Autodesk Inventor part; units mm, degrees
ref_plane "YZ Plane" through (0, 0, 0) normal (1, 0, 0) x (0, 1, 0)
ref_plane "XZ Plane" through (0, 0, 0) normal (0, 1, 0) x (-1, 0, 0)
ref_plane "XY Plane" through (0, 0, 0) normal (0, 0, 1) x (1, 0, 0)
sketch "Sketch1" plane through (0, 0, 0) normal (1, 0, 0) x (0, 1, 0)
  line L0 (9.8481, 428.814) -> (120.1519, 448.2635)
  line L1 (131.7365, 440.1519) -> (154.2135, 312.6787)
  line L2 (0, 78.3368) -> (0, 427.0775)
  line L3 (0, 417.0775) -> (0, 78.3368)
  line L4 (503.1119, 189.3047) -> (590.8645, 150.2346)
  line L5 (595.9326, 137.0318) -> (559.5861, 55.3964)
  line L6 (494.9423, 192.942) -> (494.9423, 192.942)
  line L7 (442.0149, 172.9748) -> (165.6696, 297.928)
  arc A0 (442.0149, 172.9748) -> (490.9347, 186.0198) centre (458.495, 209.4221) ccw
  arc A1 (154.2135, 312.6787) -> (165.6696, 297.928) centre (173.9096, 316.1516) ccw
  arc A2 (131.7365, 440.1519) -> (120.1519, 448.2635) centre (121.8884, 438.4154) ccw
  line L8 (9.8481, 428.814) -> (0, 417.0775)
  arc A3 (595.9326, 137.0318) -> (590.8645, 150.2346) centre (586.7972, 141.0991) ccw
  arc A4 (503.1119, 189.3047) -> (490.9347, 186.0198) centre (499.0446, 180.1692) ccw
  line L9 (9.651, 68.3429) -> (550.1017, 49.4699)
  arc A5 (550.1017, 49.4699) -> (559.5861, 55.3964) centre (550.4507, 59.4638) ccw
  arc A6 (0, 78.3368) -> (9.651, 68.3429) centre (10, 78.3368) ccw
  point P0 (0, 0)
  point P1 (0, 0)
  point P2 (130, 450)
  point P3 (156.0472, 302.2788)
  point P4 (0, 0)
  point P5 (534.922, 0)
  point P6 (600, 146.1672)
  point P7 (478.4622, 156.4947)
  point P8 (0, 427.0775)
  point P9 (537.6655, 6.1619)
  point P10 (0, 417.0775)
  dimension "d0" = 130
  dimension "d1" = 404.922
  dimension "d3" = 150
  dimension "d5" = 115
  dimension "d7" = 10
  dimension "d9" = 40
  dimension "d10" = 40
  dimension "d11" = 20
  dimension "d12" = 10
  dimension "d13" = 10
  dimension "d14" = 10
  dimension "d21" = 10
extrude "Extrusion1" add sketch "Sketch1" along normal blind 16
sketch "Sketch2" plane through (0, 0, 0) normal (-1, 0, 0) x (0, 0, 1)
  point P0 (0, 0)
sketch "Sketch3" plane through (0, 0, 0) normal (-1, 0, 0) x (0, 0, 1)
  line L0 (171.0338, 494.9772) -> (173.8576, 488.6347)
  line L1 (166.9664, 504.1126) -> (130.324, 487.7983)
  line L2 (130.324, 487.7983) -> (274.7158, 163.4898)
  line L3 (274.7158, 163.4898) -> (214.4218, 136.6452)
  line L4 (214.4218, 136.6452) -> (218.4892, 127.5097)
  line L5 (218.4892, 127.5097) -> (278.7831, 154.3544)
  line L6 (278.7831, 154.3544) -> (288.9516, 131.5158)
  line L7 (288.9516, 131.5158) -> (298.087, 135.5831)
  line L8 (298.087, 135.5831) -> (143.5268, 482.7303)
  line L9 (143.5268, 482.7303) -> (171.0338, 494.9772)
  line L10 (173.8576, 488.6347) -> (182.9931, 492.702)
  line L11 (182.9931, 492.702) -> (141.0991, 586.7972)
  line L12 (141.0991, 586.7972) -> (131.9637, 582.7298)
  line L13 (301.7603, 135.8301) -> (426.8309, 113.7768)
  line L14 (426.8309, 113.7768) -> (407.5559, 4.4631)
  line L15 (407.5559, 4.4631) -> (417.404, 2.7267)
  line L16 (417.404, 2.7267) -> (438.4154, 121.8884)
  line L17 (438.4154, 121.8884) -> (303.4968, 145.6782)
  line L18 (303.4968, 145.6782) -> (301.7603, 135.8301)
  line L19 (428.814, 9.8481) -> (417.0775, 0)
  line L20 (417.0775, 0) -> (78.3368, 0)
  line L21 (55.3964, 559.5861) -> (137.0318, 595.9326)
  arc A0 (150.2346, 590.8645) -> (137.0318, 595.9326) centre (141.0991, 586.7972) ccw
  line L22 (150.2346, 590.8645) -> (189.3047, 503.1119)
  arc A1 (186.0198, 490.9347) -> (189.3047, 503.1119) centre (180.1692, 499.0446) ccw
  arc A2 (186.0198, 490.9347) -> (172.9748, 442.0149) centre (209.4221, 458.495) ccw
  line L23 (172.9748, 442.0149) -> (297.928, 165.6696)
  arc A3 (297.928, 165.6696) -> (312.6787, 154.2135) centre (316.1516, 173.9096) ccw
  line L24 (312.6787, 154.2135) -> (440.1519, 131.7365)
  arc A4 (448.2635, 120.1519) -> (440.1519, 131.7365) centre (438.4154, 121.8884) ccw
  line L25 (448.2635, 120.1519) -> (428.814, 9.8481)
  line L26 (171.0338, 494.9772) -> (173.8576, 488.6347)
  line L27 (166.9664, 504.1126) -> (130.324, 487.7983)
  line L28 (130.324, 487.7983) -> (274.7158, 163.4898)
  line L29 (274.7158, 163.4898) -> (214.4218, 136.6452)
  line L30 (214.4218, 136.6452) -> (218.4892, 127.5097)
  line L31 (218.4892, 127.5097) -> (278.7831, 154.3544)
  line L32 (278.7831, 154.3544) -> (288.9516, 131.5158)
  line L33 (288.9516, 131.5158) -> (298.087, 135.5831)
  line L34 (298.087, 135.5831) -> (143.5268, 482.7303)
  line L35 (143.5268, 482.7303) -> (171.0338, 494.9772)
  line L36 (173.8576, 488.6347) -> (182.9931, 492.702)
  line L37 (182.9931, 492.702) -> (141.0991, 586.7972)
  line L38 (141.0991, 586.7972) -> (131.9637, 582.7298)
  line L39 (301.7603, 135.8301) -> (426.8309, 113.7768)
  line L40 (426.8309, 113.7768) -> (407.5559, 4.4631)
  line L41 (407.5559, 4.4631) -> (417.404, 2.7267)
  line L42 (417.404, 2.7267) -> (438.4154, 121.8884)
  line L43 (438.4154, 121.8884) -> (303.4968, 145.6782)
  line L44 (303.4968, 145.6782) -> (301.7603, 135.8301)
  line L45 (428.814, 9.8481) -> (417.0775, 0)
  line L46 (417.0775, 0) -> (78.3368, 0)
  line L47 (55.3964, 559.5861) -> (137.0318, 595.9326)
  arc A5 (150.2346, 590.8645) -> (137.0318, 595.9326) centre (141.0991, 586.7972) ccw
  line L48 (150.2346, 590.8645) -> (189.3047, 503.1119)
  arc A6 (186.0198, 490.9347) -> (189.3047, 503.1119) centre (180.1692, 499.0446) ccw
  arc A7 (186.0198, 490.9347) -> (172.9748, 442.0149) centre (209.4221, 458.495) ccw
  line L49 (172.9748, 442.0149) -> (297.928, 165.6696)
  arc A8 (297.928, 165.6696) -> (312.6787, 154.2135) centre (316.1516, 173.9096) ccw
  line L50 (312.6787, 154.2135) -> (440.1519, 131.7365)
  arc A9 (448.2635, 120.1519) -> (440.1519, 131.7365) centre (438.4154, 121.8884) ccw
  line L51 (448.2635, 120.1519) -> (428.814, 9.8481)
  line L52 (417.404, 2.7267) -> (438.4154, 121.8884)
  line L53 (58.3797, 539.0217) -> (136.0311, 573.5943)
  line L54 (54.3124, 548.1571) -> (141.0991, 586.7972)
  line L55 (136.0311, 573.5943) -> (131.9637, 582.7298)
  line L56 (141.0991, 586.7972) -> (182.9931, 492.702)
  line L57 (182.9931, 492.702) -> (173.8576, 488.6347)
  line L58 (166.9664, 504.1126) -> (136.0311, 573.5943)
  line L59 (166.9664, 504.1126) -> (130.324, 487.7983)
  line L60 (130.324, 487.7983) -> (274.7158, 163.4898)
  line L61 (274.7158, 163.4898) -> (214.4218, 136.6452)
  line L62 (214.4218, 136.6452) -> (218.4892, 127.5097)
  line L63 (218.4892, 127.5097) -> (278.7831, 154.3544)
  line L64 (278.7831, 154.3544) -> (288.9516, 131.5158)
  line L65 (288.9516, 131.5158) -> (298.087, 135.5831)
  line L66 (298.087, 135.5831) -> (143.5268, 482.7303)
  line L67 (143.5268, 482.7303) -> (171.0338, 494.9772)
  line L68 (171.0338, 494.9772) -> (173.8576, 488.6347)
  line L69 (303.4968, 145.6782) -> (301.7603, 135.8301)
  line L70 (301.7603, 135.8301) -> (426.8309, 113.7768)
  line L71 (426.8309, 113.7768) -> (407.5559, 4.4631)
  line L72 (407.5559, 4.4631) -> (417.404, 2.7267)
  line L73 (417.404, 2.7267) -> (438.4154, 121.8884)
  line L74 (438.4154, 121.8884) -> (303.4968, 145.6782)
  line L75 (131.9637, 582.7298) -> (54.3123, 548.1572)
  line L76 (54.3123, 548.1572) -> (58.3797, 539.0217)
  line L77 (58.3797, 539.0217) -> (136.0311, 573.5943)
  line L78 (136.0311, 573.5943) -> (166.9664, 504.1126)
  line L79 (68.3429, 9.651) -> (49.4699, 550.1017)
  arc A10 (55.3964, 559.5861) -> (49.4699, 550.1017) centre (59.4638, 550.4507) ccw
  arc A11 (68.3429, 9.651) -> (78.3368, 0) centre (78.3368, 10) ccw
  line L80 (131.9637, 582.7298) -> (54.3123, 548.1572)
  line L81 (54.3123, 548.1572) -> (58.3797, 539.0217)
  line L82 (58.3797, 539.0217) -> (136.0311, 573.5943)
  line L83 (136.0311, 573.5943) -> (166.9664, 504.1126)
  line L84 (68.3429, 9.651) -> (49.4699, 550.1017)
  arc A12 (55.3964, 559.5861) -> (49.4699, 550.1017) centre (59.4638, 550.4507) ccw
  arc A13 (68.3429, 9.651) -> (78.3368, 0) centre (78.3368, 10) ccw
  line L85 (54.3123, 548.1572) -> (58.3797, 539.0217)
  line L86 (146.0479, 199.2472) -> (155.1834, 203.3146)
  line L87 (86.038, 358.6172) -> (76.9026, 354.5499)
  line L88 (146.0479, 199.2472) -> (155.1834, 203.3146)
  line L89 (86.038, 358.6172) -> (76.9026, 354.5499)
  line L90 (86.038, 358.6172) -> (155.1834, 203.3146)
  line L91 (146.0479, 199.2472) -> (155.1834, 203.3146)
  line L92 (146.0479, 199.2472) -> (76.9026, 354.5499)
  line L93 (76.9026, 354.5499) -> (86.038, 358.6172)
  line L94 (76.9026, 354.5499) -> (146.0479, 199.2472)
  line L95 (155.1834, 203.3146) -> (86.038, 358.6172)
  line L96 (76.9026, 354.5499) -> (146.0479, 199.2472)
  line L97 (155.1834, 203.3146) -> (86.038, 358.6172)
  point P0 (0, 0)
  point P1 (131.9642, 582.73)
extrude "Extrusion2" cut sketch "Sketch3" against normal blind 7 contours L9 L8 L7 L6 L5 L4 L3 L2 L1 L58 L55 L12 L11 L10 L0 | L55 L53 L76 L54 | L18 L17 L16 L15 L14 L13 | L92 L87 L90 L86
properties part number "Arcade_Right"
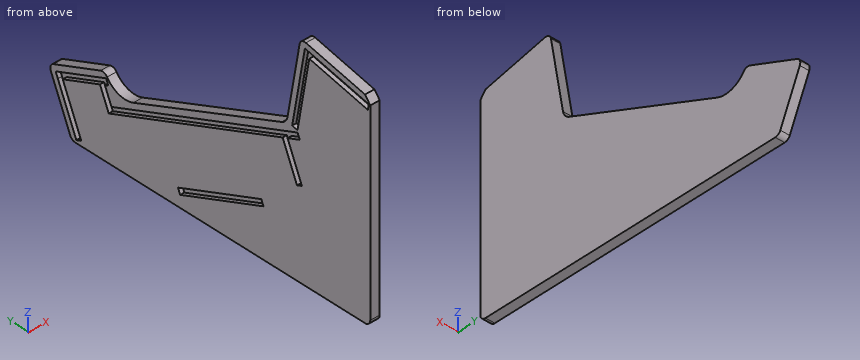
Design review of the part built by this model. Coordinates are the model's own, in mm. Give positions to 0.01 mm unless a question says otherwise; leave off trailing zeros. Loops run counter-clockwise (first coordinate to the right, second up) from the corner with the lowest first, then second, coordinate; pieces in that order, holes last. Notation, with made-up numbers: (78.5, 35) -> (101.5, 35) arc R21 ccw to (101.5, 39) -> close; hole circle Ø9 at (-21.75, -23.75). An arc over 180 degrees is marked (long way). One line per item, written item: value.
Q1. We need section B-B on y = 512.5. Give the boundary of the cut face in (x, z).
Numbers:
outline: (0, 50.78) -> (16, 50.78) -> (16, 185.12) -> (0, 185.12) -> (0, 174.18) -> (7, 174.18) -> (7, 163.23) -> (0, 163.23) -> close
Q2. For L1, parallel to Z at x = 6, y = 351; L2, parallel to Z at x = 6, y = 269.5; L3, parallel to Y at x = 6.75, z = 105.5, list the stretches that pass through material, from the lowest coordinate up.
Numbers:
L1: z = 56.42 to 78.48, 89.43 to 191.23, 202.18 to 214.13
L2: z = 59.27 to 114.77, 125.72 to 227.52, 238.46 to 250.98
L3: y = 0 to 290.32, 314.9 to 560, 570.95 to 581.89
Q3. We need section A-A on z = 251. Give the boundary of the cut face in (x, y).
Numbers:
outline: (0, 0) -> (16, 0) -> (16, 269.46) -> (0, 269.46) -> (0, 241.34) -> (7, 241.34) -> (7, 216.76) -> (0, 216.76) -> (0, 152.93) -> (7, 152.93) -> (7, 141.98) -> (0, 141.98) -> close
Q4. We need section D-D on z = 350.5. Give the boundary of the cut face in (x, y), and give its area (3 significant figures).
Numbers:
outline: (0, 0) -> (16, 0) -> (16, 147.54) -> (0, 147.54) -> (0, 137.39) -> (7, 137.39) -> (7, 127.24) -> (0, 127.24) -> close
area: 2,290 mm^2
Q5. For pin 1 Ø5 at (x, y) = (11, 333) entering from +Z; pin 2 Ø2 at (x, y) = (4.5, 94.5) entering from +Z; pin 3 Ø5 at (x, y) = (12.5, 350.5) entering from -Z, all flat-tipped, find the tip position at first contact; note any pin that passes through.
Numbers:
pin 1: stops at z = 223.4
pin 2: stops at z = 443.92
pin 3: stops at z = 56.35
Q6. We need section C-C on y = 231. Give the boundary of the cut face in (x, z), and give its area (3 significant figures).
Numbers:
outline: (0, 60.61) -> (16, 60.61) -> (16, 268.39) -> (0, 268.39) -> (0, 255.6) -> (7, 255.6) -> (7, 244.66) -> (0, 244.66) -> (0, 142.86) -> (7, 142.86) -> (7, 131.91) -> (0, 131.91) -> close
area: 3,170 mm^2
